Geometry: final body of the model. Coordinates: model frame, mm. A direction names the side the tool comes from. Give positions to 0.01 mm unless a question says otherwise; leave off trailing zeros. Loops run counter-clockwise (first coordinate to the right, second up) from the corner with the lowest first, then second, coordinate; pieces in that order, holes last.
from build123d import *

# Parameters (mm, degrees)
SKETCH1_W           = 120
SKETCH1_H           = 44
BOSS_EXTRUDE1_DEPTH = 5
SKETCH2_W           = 120
SKETCH2_H           = 5
BOSS_EXTRUDE2_DEPTH = 20
SKETCH3_R           = 5
CUT_EXTRUDE1_DEPTH  = 79.492037813
SKETCH4_R           = 5
CUT_EXTRUDE3_DEPTH  = 67.962676171


with BuildPart() as part:
    # Sketch1 → Boss-Extrude1 (new body)
    with BuildSketch(Plane(origin=(0, 0, 0), x_dir=(1, 0, 0), z_dir=(0, 1, 0))):
        Rectangle(SKETCH1_W, SKETCH1_H)
    extrude(amount=BOSS_EXTRUDE1_DEPTH)

    # Sketch2 → Boss-Extrude2 (add)
    with BuildSketch(Plane(origin=(0, 5, 0), x_dir=(1, 0, 0), z_dir=(0, 1, 0))):
        with Locations((0, 19.5)):
            Rectangle(SKETCH2_W, SKETCH2_H)
        with Locations((0, -19.5)):
            Rectangle(SKETCH2_W, SKETCH2_H)
    extrude(amount=BOSS_EXTRUDE2_DEPTH)

    # Sketch3 → Cut-Extrude1 (cut, through all)
    with BuildSketch(Plane.XY.offset(22)):
        with Locations((40, 10)):
            Circle(SKETCH3_R)
        with Locations((-40, 10)):
            Circle(SKETCH3_R)
    extrude(amount=-CUT_EXTRUDE1_DEPTH, mode=Mode.SUBTRACT)

    # Sketch4 → Cut-Extrude3 (cut, through all)
    with BuildSketch(Plane(origin=(0, 5, 0), x_dir=(1, 0, 0), z_dir=(0, 1, 0))):
        with Locations(Location((20, 10, 0), (0, 0, 270))):
            Circle(SKETCH4_R)
        with Locations(Location((20, -10, 0), (0, 0, 270))):
            Circle(SKETCH4_R)
        with Locations(Location((-20, 10, 0), (0, 0, 270))):
            Circle(SKETCH4_R)
        with Locations(Location((-20, -10, 0), (0, 0, 270))):
            Circle(SKETCH4_R)
    extrude(amount=-CUT_EXTRUDE3_DEPTH, mode=Mode.SUBTRACT)


solid = part.part
Item 1: Section query D-D on y = 10. Return loops of the section in (x, z), plus the area to 3 significant figures.
Values follow:
outline: (-60, -22) - (-45, -22) - (-45, -17) - (-60, -17) - close; (-60, 17) - (-45, 17) - (-45, 22) - (-60, 22) - close; (-35, -22) - (35, -22) - (35, -17) - (-35, -17) - close; (-35, 17) - (35, 17) - (35, 22) - (-35, 22) - close; (45, -22) - (60, -22) - (60, -17) - (45, -17) - close; (45, 17) - (60, 17) - (60, 22) - (45, 22) - close
area: 1,000 mm2
Item 2: Pin query (flat end, axial travel): pin 1 (13 mm diameter, centred on x = 20, z = -10, fed in from +Y). Return the tip coordinate at first contact, or that it passes through.
Values follow:
pin 1: stops at y = 5
Item 3: Section query C-C on z = -10. Return loops of the section in (x, y), plus the area to 3 significant figures.
Values follow:
outline: (-60, 0) - (-25, 0) - (-25, 5) - (-60, 5) - close; (-15, 0) - (15, 0) - (15, 5) - (-15, 5) - close; (25, 0) - (60, 0) - (60, 5) - (25, 5) - close
area: 500 mm2
Item 4: Section query B-B on y = 20.5. Return loops of the section in (x, z).
Values follow:
outline: (-60, -22) - (60, -22) - (60, -17) - (-60, -17) - close; (-60, 17) - (60, 17) - (60, 22) - (-60, 22) - close
Item 5: Draft query along Y for faces 1 (the face through (-1, 5, 0)), 2 (the face through (-45, 10, -19)), 3 (the face through (15.564, 2.535, 12.307)). Return one class per face: +Y half, -Y half, draft (parallel to the pull), parting line (faces both ways), or undercut.
Values follow:
face 1: +Y half
face 2: undercut
face 3: draft
Item 6: Ray query, probe 1 along X at (y, z) = (2, 10); probe 2 along X at (y, z) = (10, -18.1); probe 3 along Z at (x, y) = (32, 11.5). Return the intervals inside material, ascending.
Values follow:
probe 1: x = -60 to -25, -15 to 15, 25 to 60
probe 2: x = -60 to -45, -35 to 35, 45 to 60
probe 3: z = -22 to -17, 17 to 22
Item 7: Section query A-A on x = -20. Return loops of the section in (y, z), plus the area to 3 significant figures.
Values follow:
outline: (0, -22) - (25, -22) - (25, -17) - (5, -17) - (5, -15) - (0, -15) - close; (0, -5) - (5, -5) - (5, 5) - (0, 5) - close; (0, 15) - (5, 15) - (5, 17) - (25, 17) - (25, 22) - (0, 22) - close
area: 320 mm2
Item 8: Set-up query: faces 4 (the face through (-1, 15, -17)), 5 (the face through (-24.436, 2.535, 12.307)). Return all of +Z, -Z, +X, -X, +Y, -Y with unobstructed straight access to the full face (end or side cutting, diameter ignored); none if empty.
Values follow:
face 4: +X, -X, +Y
face 5: +Y, -Y
